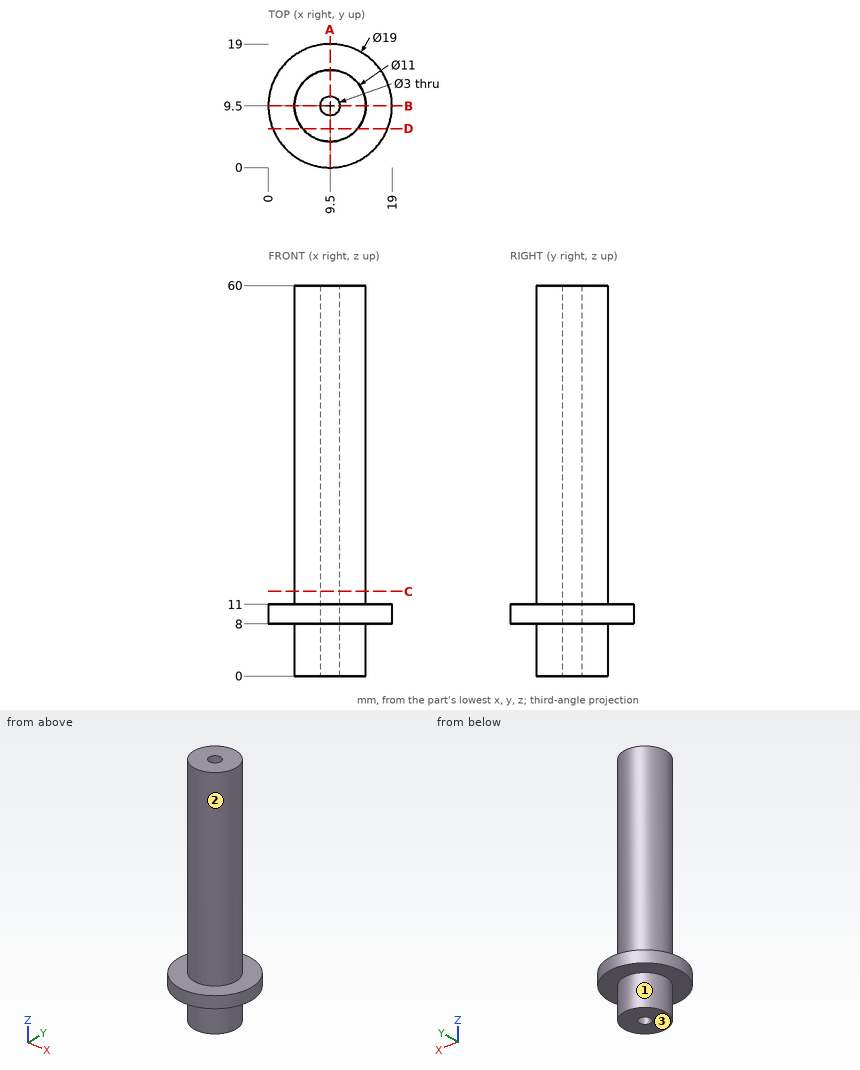
Job drawing, mm, ordinate dimensions from the low corner. One solid piece. A direction names the side the tool comes from. Round coordinates to 2 decimals unless told otherwise and drop trailing zeros. Loops run counter-clockwise (first coordinate to the right, second up) from the corner with the lowest first, then second, coordinate; pieces in that order, holes last.
(1) Cut at C-C (z = 13). Give the cut face in (x, y).
(2) Wall check: line 1 along X through (y, z) = (9.5, 41); line 2 along Z through (x, y) = (15, 7). Give the ranges that are in metal, low to high.
(3) Drop flat-ended pins along their axis: pin 1 (5 mm diameter, centred on x = 5.5, z = 47.5, fed in from +Y); pin 2 (2 mm diameter, centred on x = 8, z = 8.5, fed in from +Y); pin 3 (2 mm diameter, centred on y = 13, z = 48, fed in from -X). Give the stop position or say it passes through.
(4) Which spindle directions (+Z, -Z, +X, -X, +Y, -Y) get a long thin tool onto all of the face, cutting with end or side? Do the marked faces 1, 2 and 3. Say none if no direction does.
(5) Cut at D-D (y = 6). Give the cut face in (x, z).
(6) Cut at A-A (x = 9.5). Give the cut face in (y, z), plus the area to 3 significant figures.
Findings below:
1. outline: circle Ø11 at (9.5, 9.5); hole circle Ø3 at (9.5, 9.5)
2. line 1: x = 4 to 8, 11 to 15
2. line 2: z = 8 to 11
3. pin 1: stops at y = 14.79
3. pin 2: stops at y = 18.99
3. pin 3: stops at x = 4.6
4. face 1: -Z
4. face 2: +Z
4. face 3: -Z, +X, -X, +Y, -Y
5. outline: (0.67, 8) - (5.26, 8) - (5.26, 0) - (13.74, 0) - (13.74, 8) - (18.33, 8) - (18.33, 11) - (13.74, 11) - (13.74, 60) - (5.26, 60) - (5.26, 11) - (0.67, 11) - close
6. outline: (0, 8) - (4, 8) - (4, 0) - (8, 0) - (8, 60) - (4, 60) - (4, 11) - (0, 11) - close; (11, 0) - (15, 0) - (15, 8) - (19, 8) - (19, 11) - (15, 11) - (15, 60) - (11, 60) - close
6. area: 504 mm2
